Source: CAD feature listing. Evaluate the final solid. Frame: model axes, mm. A direction names the side the tool comes from. Give positions to 0.01 mm unless a question says otherwise; leave off trailing zeros. Loops run counter-clockwise (first coordinate to the right, second up) from the corner with the lowest first, then second, coordinate; pieces in that order, holes last. Notation, with made-up numbers: (-28, 14) -> (-18, 14) arc R20 ccw to (-18, 22) -> close; hole circle Ø5 at (-16.5, 22). An arc over 180 degrees is marked (long way). Return JSON: item names as keys, results as strings. Group by question number.
(1) Draft query along X for faces 1 (the face through (-24, -11, -81.28)), 2 (the face through (48.94, 15.41, -40.07)), 3 (the face through (105, 48, 12)). Return one class per face: released by +X, released by -X, zero draft, split by the parting line, or undercut.
(2) Cut plane A-A on x = 0. Return loops of the section in (y, z), then the cut area to 3 significant figures.
(3) Cut plane D-D on z = -71.5. Return loops of the section in (x, y).
(4) Ray query, line 1 (Z direction, x = -39, y = 82.5); line 2 (Z direction, x = 26, y = 18); line 3 (X direction, y = 38, z = -14). Return the intervals inside material, ascending. Write a range as from..to.
(5) Pin query (flat end, axial travel): pin 1 (6 mm diameter, centred on x = -24.5, z = -32, fed in from -Y); pin 2 (12 mm diameter, centred on x = 10.5, y = 75.5, fed in from -Z); pin 3 (3 mm diameter, centred on x = -8, z = -60, fed in from +Y); pin 4 (7.5 mm diameter, centred on x = -44.36, y = -107.1, fed in from +Z). Return the tip coordinate at first contact, or that it passes through.
(6) Cut plane C-C on z = 17.5. Give the number of separate pieces and of enclosed holes in the cut face, then the cut area to 3 significant figures.
(7) Access query for faces 4 (the face through (68.96, -95.85, 12.43)), 5 (the face through (55, 2, 0)), 6 (the face through (-6.349, 48.353, -26.392)). Directions: +Z, -Z, +X, -X, +Y, -Y. A direction counts if a zero-diameter tool reaches every point of the face in a straight line with its end or side. Return the directions, or none.
```python
from build123d import *

# Parameters (mm, degrees)
SKETCH1_R          = 51.308
SKETCH1_R_2        = 48.768
EXTRUDE1_DEPTH     = 81.28
EXTRUDE2_START     = 24.511
SKETCH2_R          = 127
SKETCH2_R_2        = 48.768
EXTRUDE2_DEPTH     = 24.511
CUT_EXTRUDE1_REACH = 210.446
SKETCH3_R          = 4.2
CIRPATTERN1_COUNT  = 24
EXTRUDE3_START     = -2.54
SKETCH4_R          = 51.308
SKETCH4_R_2        = 25.4
EXTRUDE3_DEPTH     = 2.54


with BuildPart() as part:
    # Sketch1 → Extrude1 (new body)
    with BuildSketch(Plane.XY):
        Circle(SKETCH1_R)
        Circle(SKETCH1_R_2, mode=Mode.SUBTRACT)
    extrude(amount=-EXTRUDE1_DEPTH)

    # Sketch2 → Extrude2 (add)
    with BuildSketch(Plane.XY.offset(EXTRUDE2_START)):
        Circle(SKETCH2_R)
        Circle(SKETCH2_R_2, mode=Mode.SUBTRACT)
    extrude(amount=-EXTRUDE2_DEPTH)

    # Sketch3 → Cut-Extrude1 (cut, up to next)
    with BuildSketch(Plane.XY.offset(24.511), mode=Mode.PRIVATE) as cut_extrude1_sk1:
        with Locations((15.131327149, -114.933840422)):
            Circle(SKETCH3_R)
    cut_extrude1_tool1 = extrude(cut_extrude1_sk1.sketch, amount=-CUT_EXTRUDE1_REACH, mode=Mode.PRIVATE) & part.part
    cut_extrude1 = cut_extrude1_tool1.solids().sort_by_distance((15.131327, -114.93384, 24.511))[0]
    add(cut_extrude1, mode=Mode.SUBTRACT)

    # CirPattern1: Cut-Extrude1 ×24 about axis
    cirpattern1_axis = Axis((0, 0, 0), (0, 0, 1))
    for i in range(1, CIRPATTERN1_COUNT):
        add(cut_extrude1.rotate(cirpattern1_axis, i * 360 / CIRPATTERN1_COUNT), mode=Mode.SUBTRACT)

    # Sketch4 → Extrude3 (add)
    with BuildSketch(Plane(origin=(0, 0, -81.28), x_dir=(-1, 0, 0), z_dir=(0, 0, -1)).offset(EXTRUDE3_START)):
        with Locations(Location((0, 0, 0), (0, 0, 180))):
            Circle(SKETCH4_R)
        Circle(SKETCH4_R_2, mode=Mode.SUBTRACT)
    extrude(amount=EXTRUDE3_DEPTH)


solid = part.part
```
Answers:
{
 "1": {"face 1": "zero draft", "face 2": "split by the parting line", "face 3": "undercut"},
 "2": {"outline": "(-127, 0) -> (-51.31, 0) -> (-51.31, -81.28) -> (-25.4, -81.28) -> (-25.4, -78.74) -> (-48.77, -78.74) -> (-48.77, 24.51) -> (-127, 24.51) -> close; (25.4, -81.28) -> (51.31, -81.28) -> (51.31, 0) -> (127, 0) -> (127, 24.51) -> (48.77, 24.51) -> (48.77, -78.74) -> (25.4, -78.74) -> close", "area": "4,370 mm²"},
 "3": {"outline": "circle Ø102.62 at (0, 0); hole circle Ø97.54 at (0, 0)"},
 "4": {"line 1": "0..24.51", "line 2": "-81.28..-78.74", "line 3": "-34.47..-30.57, 30.57..34.47"},
 "5": {"pin 1": "y = -46.59", "pin 2": "z = 0", "pin 3": "y = 50.89", "pin 4": "through"},
 "6": {"separate pieces": "1", "enclosed holes": "25", "area": "41,900 mm²"},
 "7": {"face 4": "+Z, -Z", "face 5": "-Z", "face 6": "+Z"}
}
